from build123d import *

# Parameters (mm, degrees)
SKETCH2_W                = 20
SKETCH2_H                = 5
BOSS_EXTRUDE2_DEPTH      = 25
BOSS_EXTRUDE3_DEPTH      = 5
BOSS_EXTRUDE3_DEPTH_BACK = 25
SKETCH3_W                = 5
SKETCH3_H                = 5
SKETCH4_W                = 25
SKETCH4_H                = 5
BOSS_EXTRUDE4_DEPTH      = 25
SKETCH5_R                = 7
CUT_EXTRUDE1_DEPTH       = 30
CUT_EXTRUDE2_DEPTH       = 10
SKETCH7_W                = 5
SKETCH7_H                = 5
BOSS_EXTRUDE5_DEPTH      = 7


with BuildPart() as part:
    # Sketch2 → Boss-Extrude2 (new body)
    with BuildSketch(Plane.XY):
        with Locations((15, 2.5)):
            Rectangle(SKETCH2_W, SKETCH2_H)
    extrude(amount=BOSS_EXTRUDE2_DEPTH)

    # Sketch3 → Boss-Extrude3 (add, two sides: drawn at the far end of the back side and taken through both)
    with BuildSketch(Plane(origin=(0, 0, 0), x_dir=(-1, 0, 0), z_dir=(0, 0, -1)).offset(-BOSS_EXTRUDE3_DEPTH_BACK)):
        with Locations((-2.5, 2.5)):
            Rectangle(SKETCH3_W, SKETCH3_H)
    extrude(amount=BOSS_EXTRUDE3_DEPTH + BOSS_EXTRUDE3_DEPTH_BACK)

    # Sketch4 → Boss-Extrude4 (add)
    with BuildSketch(Plane(origin=(0, 0, -5), x_dir=(-1, 0, 0), z_dir=(0, 0, -1))):
        with Locations((-12.5, 2.5)):
            Rectangle(SKETCH4_W, SKETCH4_H)
    extrude(amount=BOSS_EXTRUDE4_DEPTH)

    # Sketch5 → Cut-Extrude1 (cut)
    with BuildSketch(Plane(origin=(0, 5, 0), x_dir=(1, 0, 0), z_dir=(0, 1, 0))):
        with Locations(Location((15, -10.5, 0), (0, 0, 180))):
            Circle(SKETCH5_R)
        with Locations(Location((15, 15.5, 0), (0, 0, 180))):
            Circle(SKETCH5_R)
    extrude(amount=-CUT_EXTRUDE1_DEPTH, mode=Mode.SUBTRACT)

    # Sketch6 → Cut-Extrude2 (cut)
    with BuildSketch(Plane.XZ):
        with BuildLine():
            ThreePointArc((22.588137581, -5), (23.386954562, -10.385878866), (25, -15.586252328))
            Line((25, -15.586252328), (25, -5))
            Line((25, -5), (22.588137581, -5))
        make_face()
        with BuildLine():
            Line((25, 0), (25, 10.586252328))
            ThreePointArc((25, 10.586252328), (23.386954562, 5.385878866), (22.588137581, 0))
            Line((22.588137581, 0), (25, 0))
        make_face()
    extrude(amount=-CUT_EXTRUDE2_DEPTH, mode=Mode.SUBTRACT)

    # Sketch7 → Boss-Extrude5 (add)
    with BuildSketch(Plane(origin=(5, 0, 0), x_dir=(0, 0, -1), z_dir=(1, 0, 0))):
        with Locations((2.5, 2.5)):
            Rectangle(SKETCH7_W, SKETCH7_H)
    extrude(amount=BOSS_EXTRUDE5_DEPTH)


solid = part.part
Verification items for the finished model (mm, model axes). A direction names the side the tool comes from. Give positions to 0.01 mm unless a question says otherwise; leave off trailing zeros. Order: outer loops, then holes, each group sorted by start corner. A loop starts at its lowest first (then second) coordinate and runs counter-clockwise, first axis right, second up. Notation, with made-up numbers: M 22,-24.75 L 41,-24.75 A18 cw 41,0.25 Z; hole C 28,-11.5 d3. An arc over 180 degrees is marked long. Answer as a JSON object with one key per item and string values. Group by question number.
1) Cross-section at A-A (x = 15). Enter the section's corners in (y, z), then the cut area to 3 significant figures.
2) Depth check by flat-ended pin: pin 1 Ø10 at (x, z) = (4.5, 18) entering from -Y. Enter the tip coordinate at first touch or a pass-through.
3) Scan lines: line 1 along Z through (x, y) = (15, 1.5); line 2 along Z through (x, y) = (13.5, 1.25); line 3 along X through (y, z) = (1.95, -2). Record each from-to range of solid material in increasing order. Write a range as [from, to].
4) Cross-section at D-D (z = 5). Enter the section's corners in (x, y).
5) Cross-section at B-B (y = 4.3). Enter the section's corners in (x, z).
6) Access from +Z, -Z, +X, -X, +Y, -Y to the whole of each face (thin tool, end or side, straight path). Record for faces 5 (the face through (17, 3, -5)), 6 (the face through (13, 3, 25)).
7) Mould release check, pull along X, two halves, no side actions. Record for faces 1 (the face through (10, 5, -2)), 2 (the face through (23.404, 2.465, 5.46)), 3 (the face through (21.993, 2.535, 10.808)), 4 (the face through (0, 2, -2)): released by +X, released by -X, zero draft, split by the parting line, or undercut.
8) Cross-section at C-C (z = -15). Enter the section's corners in (x, y).
Result sheet:
{
 "1": {"outline": "M 0,-30 L 5,-30 L 5,-22.5 L 0,-22.5 Z; M 0,-8.5 L 5,-8.5 L 5,-5 L 0,-5 Z; M 0,0 L 5,0 L 5,3.5 L 0,3.5 Z; M 0,17.5 L 5,17.5 L 5,25 L 0,25 Z", "area": "110 mm2"},
 "2": {"pin 1": "stops at y = 0"},
 "3": {"line 1": "z = [-30, -22.5], [-8.5, -5], [0, 3.5], [17.5, 25]", "line 2": "z = [-30, -22.34], [-8.66, -5], [0, 3.66], [17.34, 25]", "line 3": "x = [0, 12]"},
 "4": {"outline": "M 0,0 L 10.67,0 L 10.67,5 L 0,5 Z; M 19.33,0 L 23.3,0 L 23.3,5 L 19.33,5 Z"},
 "5": {"outline": "M 0,-30 L 25,-30 L 25,-15.59 A35.5 cw 22.59,-5 L 12,-5 L 12,0 L 22.59,0 A35.5 cw 25,10.59 L 25,25 L 0,25 Z; hole C 15,-15.5 d14; hole C 15,10.5 d14"},
 "6": {"face 5": "+X, +Y, -Y", "face 6": "+Z, +X, -X, +Y, -Y"},
 "7": {"face 1": "zero draft", "face 2": "released by +X", "face 3": "undercut", "face 4": "released by -X"},
 "8": {"outline": "M 0,0 L 8.02,0 L 8.02,5 L 0,5 Z; M 21.98,0 L 24.77,0 L 24.77,5 L 21.98,5 Z"}
}
